Answer from the drawing. Dimensions are ordinates in mm from the lowest x, y and z of the part. A direction names the side the tool comes from. Give positions to 0.01 mm unless a question says otherwise; leave off trailing zeros. Order: outer loops, then holes, each group sorted by start corner. A loop starts at its lowest first (then second) coordinate and runs counter-clockwise, first axis right, second up. Notation, with made-up numbers: (5, 69) - (64, 69) arc R15 cw to (64, 82) - close; hole circle Ø10 at (-27.75, -17.75). An arc over 180 degrees is marked (long way). Write each question's results on one line, items separated by ' | '.
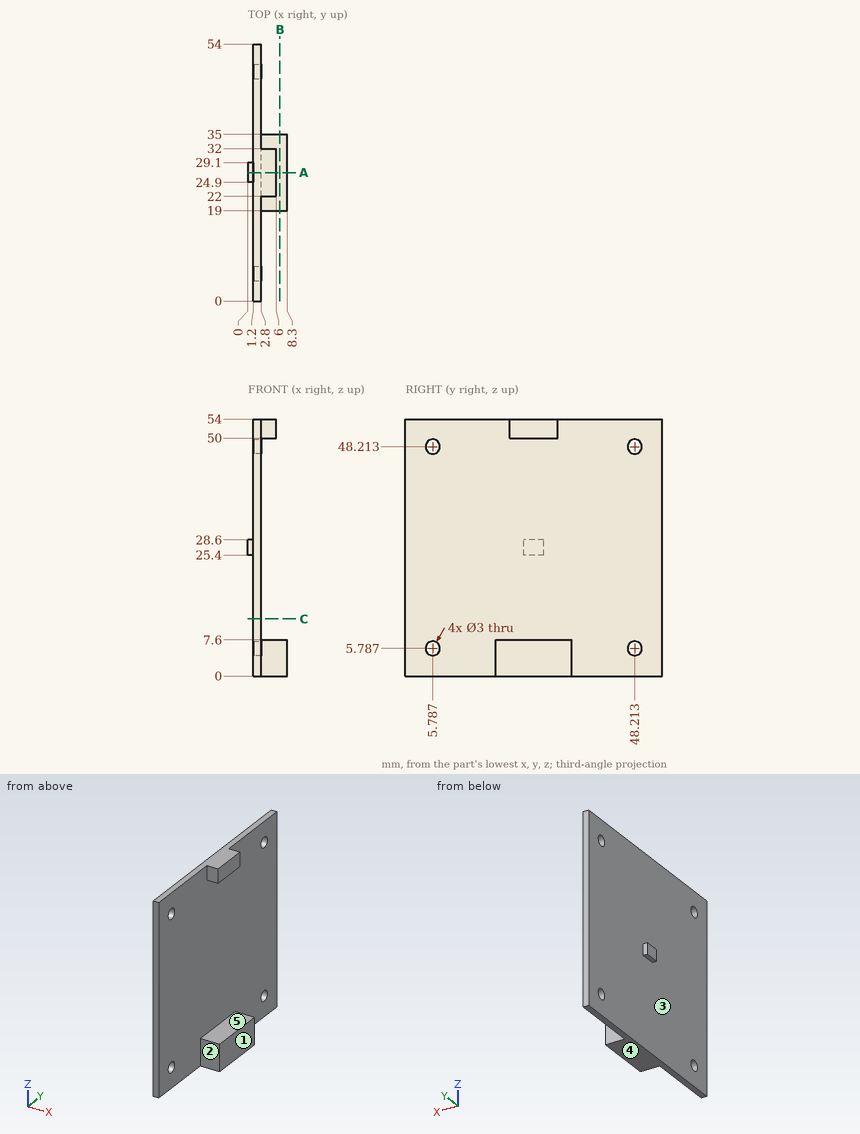
1. A cutting plane is placed at B-B, the plane x = 6.75. Write down the section's boundary in (y, z).
Answer list:
outline: (19, 0) - (35, 0) - (35, 7.6) - (19, 7.6) - close
2. Given P1, Ø10, axis at y = 13.5, z = 44.5, coming from the -X side; P2, Ø3, axis at x = 6, z = 4, coming from the +Y side; P3, Ø4, axis at y = 5.79, z = 48.21, coming from the +X side, each flat-ended and moving along its own axis, determine where each tip first touches the part or whether it passes through.
Answer list:
P1: x = 1.2 | P2: y = 35 | P3: x = 2.8
3. A cutting plane is placed at C-C, the plane z = 12. Write down the section's boundary in (x, y), then the cut area to 3 significant figures.
Answer list:
outline: (1.2, 0) - (2.8, 0) - (2.8, 54) - (1.2, 54) - close | area: 86.4 mm^2
4. Determine the mould class of the marked faces 3, 4 and 5 for opening direction Z: +Z half, -Z half, draft (parallel to the pull), parting line (faces both ways), or undercut.
Answer list:
face 3: draft | face 4: -Z half | face 5: undercut
5. Straight lines are drawn through the part: line 1 (Z direction, x = 5.75, y = 30.5); line 2 (Y direction, x = 2.5, z = 7) (1 decimal); line 3 (X direction, y = 14, z = 6). For each, find the intervals that lie inside material, in ascending order. Write a range as [from, to].
Answer list:
line 1: [0, 7.6], [50, 54] | line 2: [0, 4.9], [6.7, 47.3], [49.1, 54] | line 3: [1.2, 2.8]
6. A cutting plane is placed at A-A, the plane y = 27. Write down the section's boundary in (x, z), then the cut area to 3 significant figures.
Answer list:
outline: (0, 25.4) - (1.2, 25.4) - (1.2, 0) - (8.3, 0) - (8.3, 7.6) - (2.8, 7.6) - (2.8, 50) - (6, 50) - (6, 54) - (1.2, 54) - (1.2, 28.6) - (0, 28.6) - close | area: 145 mm^2
7. A tool of negligible diameter and unlimited length cuts with its end or side. For the marked faces 1 and 2, from which of +Z, -Z, +X, -X, +Y, -Y can it reach the whole face along a straight path? Write none if from no direction.
Answer list:
face 1: +Z, -Z, +X, +Y, -Y | face 2: +Z, -Z, +X, -Y
